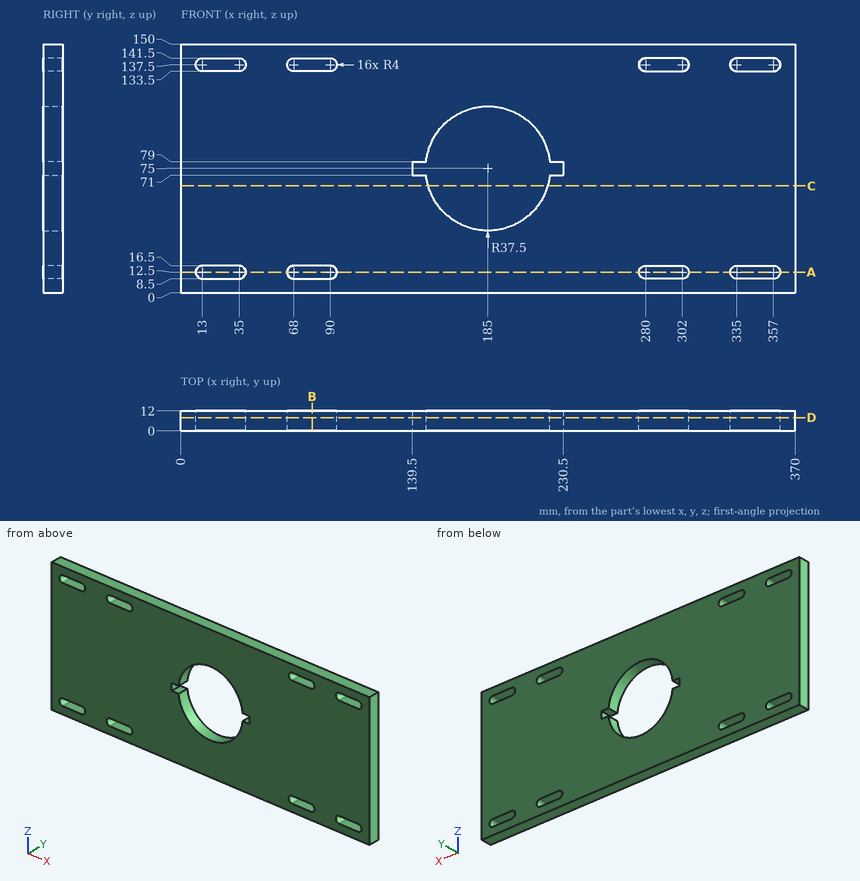
The drawing under review shows one solid part. Ordinate dimensions are in mm from its lowest x, y, z. Round coordinates to 2 decimals unless told otherwise and drop trailing zeros. Write each loop counter-clockwise with the first axis right and the second up, starting at its lowest first coordinate (ties: lowest second). Pieces come first, ordered by that corner, then holes.
(1) We need section B-B on x = 79. Give the boundary of the cut face in (y, z), and give its area (3 significant figures).
(2) We need section C-C on z = 64.5. Give the boundary of the cut face in (x, y).
(3) We need section D-D on y = 8. Give the number of separate pieces and of enclosed holes in the cut face, and give its area (3 significant figures).
(4) Wall thickness on L1, parallel to Z at x = 295, y = 5; L2, parallel to X at y = 1, z = 12; L3, parallel to Z at x = 225.5, y = 6.5: over which ranges is each line inside the solid? List them lowest first.
(5) We need section A-A on z = 12.5. Give the boundary of the cut face in (x, y).
Findings below:
1. outline: (0, 0) - (12, 0) - (12, 8.5) - (0, 8.5) - close; (0, 16.5) - (12, 16.5) - (12, 133.5) - (0, 133.5) - close; (0, 141.5) - (12, 141.5) - (12, 150) - (0, 150) - close
1. area: 1,610 mm2
2. outline: (0, 0) - (149, 0) - (149, 12) - (0, 12) - close; (221, 0) - (370, 0) - (370, 12) - (221, 12) - close
3. separate pieces: 1
3. enclosed holes: 9
3. area: 49,100 mm2
4. L1: z = 0 to 8.5, 16.5 to 133.5, 141.5 to 150
4. L2: x = 0 to 9.03, 38.97 to 64.03, 93.97 to 276.03, 305.97 to 331.03, 360.97 to 370
4. L3: z = 0 to 71, 79 to 150
5. outline: (0, 0) - (9, 0) - (9, 12) - (0, 12) - close; (39, 0) - (64, 0) - (64, 12) - (39, 12) - close; (94, 0) - (276, 0) - (276, 12) - (94, 12) - close; (306, 0) - (331, 0) - (331, 12) - (306, 12) - close; (361, 0) - (370, 0) - (370, 12) - (361, 12) - close
